CAD build for the part. Positions are in the model's coordinates, mm. A direction names the side the tool comes from. Round coordinates to 2 decimals unless told otherwise and drop trailing zeros. Write each loop counter-clockwise with the first axis right and the second up, starting at its lowest first coordinate (ties: lowest second). Pieces come first, ordered by that corner, then holes. Notation, with made-up numbers: (-12, 18) -> (40, 18) arc R7 ccw to (40, 25) -> close; hole circle Ø2 at (-39, 13). An arc over 180 degrees is marked (long way). Put each result on its own line as item: value. Start each with the question number.
1. Saw through at B-B on x = 2.75. List the corners of the cut face in (y, z).
2. Saw through at D-D on z = 4.25. List the corners of the cut face in (x, y).
3. 3-axis set-ups, long thin cutter, end or side, ignore diameter. For faces 1 (the flat face through (6, 0.905, 17)), 2 (the flat face through (-5, 0, 2.1)), 3 (the flat face through (0, 3.2, 8)), 4 (the flat face through (-4.95, 6, 17)), 5 (the flat face through (0, -5, 15.848)): which of +Z, -Z, +X, -X, +Y, -Y reach the whole face in a straight line?
4. Pull direction Y, two halves, no side cores. Call faces 6 (the flat face through (0, -5, 1.6)), 7 (the flat face through (4.95, 2, 17)), 8 (the flat face through (0, -3.8, 9)): pulls with the +Y half, pulls with the -Y half, needs draft (parallel to the pull), parting line crosses it, or undercut.
5. Saw through at A-A on y = 1.75. List the corners of the cut face in (x, z).
6. Drill centre lines: line 1 (Y direction, x = -3, z = 6); line 2 (Z direction, x = 3.75, y = 8.25); line 3 (Y direction, x = -3, z = 1.75). Where is each one in solid material? Low to high. Write a range as from..to.
7. Flat gauge pins, fed straight in: P1, Ø1.5, axis at x = -4.5, y = 2, coming from the +Z side; P2, Ø3, axis at x = -0.5, y = 6.5, coming from the +Z side; P3, Ø1.7, axis at y = -9, z = 1, coming from the +X side. Where does each tip first touch, or does it go through?
8. Saw through at C-C on x = 6.25. List the corners of the cut face in (y, z) (3 decimals).
from build123d import *

# Parameters (mm, degrees)
F0_W           = 13.9
F0_H           = 22
F1_DEPTH       = 19.8
F4_W           = 13.9
F4_H           = 22
F4_W_2         = 7.6
F4_H_2         = 7.6
F5_DEPTH       = 13.1
F6_W           = 6.4
F6_H           = 6.4
F7_DEPTH       = 19.801
F8_W           = 2.1
F8_H           = 22
F8_W_2         = 6.1
F9_DEPTH       = 1.6
F10_W          = 2.1
F10_H          = 4.05
F10_W_2        = 6.1
F11_DEPTH      = 0.5
F12_W          = 6.1
F12_H          = 4.05
F12_W_2        = 2
F12_H_2        = 2
F13_DEPTH      = 4.6
F14_W          = 6.4
F14_H          = 3.9517926995
F15_DEPTH      = 11.001
F15_DEPTH_BACK = 11.001
F16_R          = 0.225
F17_DEPTH      = 5.5
F18_W          = 2
F18_H          = 0.5
F19_DEPTH      = 2


with BuildPart() as f1:
    # F0 (on Top) → F1 (new body)
    with BuildSketch(Plane.XY):
        Rectangle(F0_W, F0_H)
    extrude(amount=F1_DEPTH)

    # F4 (on offset) → F5 (cut, through all)
    with BuildSketch(Plane(origin=(0, 0, 2.1), x_dir=(1, 0, 0), z_dir=(0, 0, -1))):
        Rectangle(F4_W, F4_H)
        Rectangle(F4_W_2, F4_H_2, mode=Mode.SUBTRACT)
    extrude(amount=-F5_DEPTH, mode=Mode.SUBTRACT)

    # F6 (on face) → F7 (cut, through all)
    with BuildSketch(Plane.XY.offset(19.8)):
        Rectangle(F6_W, F6_H)
    extrude(amount=-F7_DEPTH, mode=Mode.SUBTRACT)

    # F8 (on face) → F9 (cut)
    with BuildSketch(Plane(origin=(0, 0, 0), x_dir=(1, 0, 0), z_dir=(0, 0, -1))):
        with Locations((-5.9, 0)):
            Rectangle(F8_W, F8_H)
        Rectangle(F8_W_2, F8_H)
        with Locations((5.9, 0)):
            Rectangle(F8_W, F8_H)
    extrude(amount=-F9_DEPTH, mode=Mode.SUBTRACT)

    # F10 (on face) → F11 (cut, through all)
    with BuildSketch(Plane.XY.offset(2.1)):
        with Locations((5.9, 8.975)):
            Rectangle(F10_W, F10_H)
        with Locations((5.9, -8.975)):
            Rectangle(F10_W, F10_H)
        with Locations((0, -8.975)):
            Rectangle(F10_W_2, F10_H)
        with Locations((-5.9, -8.975)):
            Rectangle(F10_W, F10_H)
        with Locations((-5.9, 8.975)):
            Rectangle(F10_W, F10_H)
        with Locations((0, 8.975)):
            Rectangle(F10_W_2, F10_H)
    extrude(amount=-F11_DEPTH, mode=Mode.SUBTRACT)

    # F12 (on face) → F13 (cut, through all)
    with BuildSketch(Plane(origin=(0, 0, 15.2), x_dir=(1, 0, 0), z_dir=(0, 0, -1))):
        with Locations((0, -8.975)):
            Rectangle(F12_W, F12_H)
        with Locations((5.95, -5.715)):
            Rectangle(F12_W_2, F12_H_2)
        with Locations((5.95, -1.905)):
            Rectangle(F12_W_2, F12_H_2)
        with Locations((5.95, 1.905)):
            Rectangle(F12_W_2, F12_H_2)
        with Locations((5.95, 5.715)):
            Rectangle(F12_W_2, F12_H_2)
        with Locations((-5.95, 5.715)):
            Rectangle(F12_W_2, F12_H_2)
        with Locations((0, 8.975)):
            Rectangle(F12_W, F12_H)
        with Locations((-5.95, 1.905)):
            Rectangle(F12_W_2, F12_H_2)
        with Locations((-5.95, -1.905)):
            Rectangle(F12_W_2, F12_H_2)
        with Locations((-5.95, -5.715)):
            Rectangle(F12_W_2, F12_H_2)
    extrude(amount=-F13_DEPTH, mode=Mode.SUBTRACT)

    # F14 (on Front) → F15 (cut, two sides)
    with BuildSketch(Plane.XZ) as f15_sk:
        with Locations((0, 17.8241036503)):
            Rectangle(F14_W, F14_H)
    extrude(amount=-F15_DEPTH, mode=Mode.SUBTRACT)
    extrude(f15_sk.sketch, amount=F15_DEPTH_BACK, mode=Mode.SUBTRACT)

    # F16 (on face) → F17 (join)
    with BuildSketch(Plane.XY.offset(19.8)):
        with Locations((5.08, 7.62)):
            Circle(F16_R)
        with Locations((5.08, 3.81)):
            Circle(F16_R)
        with Locations((5.08, 0)):
            Circle(F16_R)
        with Locations((5.08, -3.81)):
            Circle(F16_R)
        with Locations((5.08, -7.62)):
            Circle(F16_R)
        with Locations((-5.08, -7.62)):
            Circle(F16_R)
        with Locations((-5.08, -3.81)):
            Circle(F16_R)
        with Locations((-5.08, 0)):
            Circle(F16_R)
        with Locations((-5.08, 3.81)):
            Circle(F16_R)
        with Locations((-5.08, 7.62)):
            Circle(F16_R)
    extrude(amount=F17_DEPTH)

    # F18 (on face) → F19 (join)
    with BuildSketch(Plane.XY.offset(19.8)):
        with Locations((-5.95, 10.75)):
            Rectangle(F18_W, F18_H)
        with Locations((-5.95, -10.75)):
            Rectangle(F18_W, F18_H)
        with Locations((5.95, -10.75)):
            Rectangle(F18_W, F18_H)
        with Locations((5.95, 10.75)):
            Rectangle(F18_W, F18_H)
    extrude(amount=F19_DEPTH)


solid = f1.part
Return value:
1. outline: (-6.95, 1.6) -> (-3.2, 1.6) -> (-3.2, 15.85) -> (-6.95, 15.85) -> (-6.95, 15.2) -> (-3.8, 15.2) -> (-3.8, 2.1) -> (-6.95, 2.1) -> close; (3.2, 1.6) -> (6.95, 1.6) -> (6.95, 2.1) -> (3.8, 2.1) -> (3.8, 15.2) -> (6.95, 15.2) -> (6.95, 15.85) -> (3.2, 15.85) -> close
2. outline: (-3.8, -3.8) -> (3.8, -3.8) -> (3.8, 3.8) -> (-3.8, 3.8) -> close; hole (-3.2, -3.2) -> (3.2, -3.2) -> (3.2, 3.2) -> (-3.2, 3.2) -> close
3. face 1: +Z, +X
3. face 2: none
3. face 3: +Z, -Z
3. face 4: +Z, -X
3. face 5: +Z, +Y, -Y
4. face 6: needs draft
4. face 7: undercut
4. face 8: pulls with the -Y half
5. outline: (-6.95, 1.6) -> (-4.85, 1.6) -> (-4.85, 0) -> (-3.2, 0) -> (-3.2, 19.8) -> (-4.95, 19.8) -> (-4.95, 15.2) -> (-3.8, 15.2) -> (-3.8, 2.1) -> (-6.95, 2.1) -> close; (3.2, 0) -> (4.85, 0) -> (4.85, 1.6) -> (6.95, 1.6) -> (6.95, 2.1) -> (3.8, 2.1) -> (3.8, 15.2) -> (4.95, 15.2) -> (4.95, 19.8) -> (3.2, 19.8) -> close
6. line 1: y = -3.8..-3.2, 3.2..3.8
6. line 2: z = 0..2.1, 15.2..19.8
6. line 3: y = -6.95..-3.2, 3.2..6.95
7. P1: stops at z = 19.8
7. P2: stops at z = 15.85
7. P3: stops at x = 4.85
8. outline: (-11, 15.2) -> (-6.715, 15.2) -> (-6.715, 19.8) -> (-10.5, 19.8) -> (-10.5, 21.8) -> (-11, 21.8) -> close; (-6.95, 1.6) -> (6.95, 1.6) -> (6.95, 2.1) -> (-6.95, 2.1) -> close; (-4.715, 15.2) -> (-2.905, 15.2) -> (-2.905, 19.8) -> (-4.715, 19.8) -> close; (-0.905, 15.2) -> (0.905, 15.2) -> (0.905, 19.8) -> (-0.905, 19.8) -> close; (2.905, 15.2) -> (4.715, 15.2) -> (4.715, 19.8) -> (2.905, 19.8) -> close; (6.715, 15.2) -> (11, 15.2) -> (11, 21.8) -> (10.5, 21.8) -> (10.5, 19.8) -> (6.715, 19.8) -> close
